The listing builds one solid part. Answer for the finished solid, in the listing's coordinates (mm). Face numbers are marked on the shaded views. Round coordinates to 2 decimals unless told otherwise and drop trailing zeros. Write each loop counter-clockwise with the first axis right and the second up, starting at its lowest first coordinate (ties: lowest second). Pieces come first, ordered by that corner, then holes.
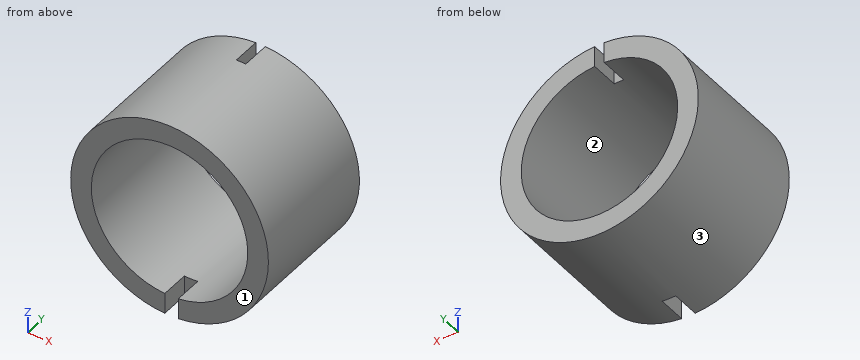
from build123d import *

# Parameters (mm, degrees)
SKETCH1_R           = 13.208
SKETCH1_R_2         = 10.45
BOSS_EXTRUDE1_DEPTH = 17.78
SKETCH2_W           = 1.27
SKETCH2_H           = 3.587114975
CUT_EXTRUDE1_DEPTH  = 3.81
SKETCH3_W           = 1.806448
SKETCH3_H           = 4.299301561
CUT_EXTRUDE2_DEPTH  = 3.81


with BuildPart() as part:
    # Sketch1 → Boss-Extrude1 (new body)
    with BuildSketch(Plane(origin=(0, 0, 0), x_dir=(1, 0, 0), z_dir=(0, 1, 0))):
        with Locations(Location((0, 0, 0), (0, 0, 270))):
            Circle(SKETCH1_R)
        with Locations(Location((0, 0, 0), (0, 0, 270))):
            Circle(SKETCH1_R_2, mode=Mode.SUBTRACT)
    extrude(amount=BOSS_EXTRUDE1_DEPTH)

    # Sketch2 → Cut-Extrude1 (cut)
    with BuildSketch(Plane(origin=(0, 17.78, 0), x_dir=(1, 0, 0), z_dir=(0, 1, 0))):
        with Locations((0, -11.851276013)):
            Rectangle(SKETCH2_W, SKETCH2_H)
    extrude(amount=-CUT_EXTRUDE1_DEPTH, mode=Mode.SUBTRACT)

    # Sketch3 → Cut-Extrude2 (cut)
    with BuildSketch(Plane.XZ):
        with Locations((0.268224, -12.348416978)):
            Rectangle(SKETCH3_W, SKETCH3_H)
    extrude(amount=-CUT_EXTRUDE2_DEPTH, mode=Mode.SUBTRACT)


solid = part.part
1. Section A-A on x = 0 is taken. Determine the outline of the cut face in (y, z), plus the area to 3 significant figures.
Geometry says:
outline: (0, 10.45) - (13.97, 10.45) - (13.97, 13.21) - (0, 13.21) - close; (3.81, -13.21) - (17.78, -13.21) - (17.78, -10.45) - (3.81, -10.45) - close
area: 77.1 mm2
2. Section C-C on z = -11 is taken. Determine the outline of the cut face in (x, y) (3 decimals).
Geometry says:
outline: (-7.311, 0) - (-0.635, 0) - (-0.635, 3.81) - (1.171, 3.81) - (1.171, 0) - (7.311, 0) - (7.311, 17.78) - (-7.311, 17.78) - close
3. Section B-B on z = 0 is taken. Determine the outline of the cut face in (x, y).
Geometry says:
outline: (-13.21, 0) - (-10.45, 0) - (-10.45, 17.78) - (-13.21, 17.78) - close; (10.45, 0) - (13.21, 0) - (13.21, 17.78) - (10.45, 17.78) - close
4. Given pin 1 (1.4 mm diameter, centred on y = 16, z = 11.5, fed in from +X); pin 2 (2 mm diameter, centred on y = 1, z = -12, fed in from -X); pin 3 (0.8 mm diameter, centred on y = 15.5, z = 11.5, fed in from -X), each flat-ended and moving along its own axis, determine where each tip first touches the part or whether it passes through.
Geometry says:
pin 1: stops at x = 7.6
pin 2: stops at x = -7.31
pin 3: stops at x = -7.16
5. For a pull along Z with two mould halves and no side action, classify the marked faces 1, 2 and 3 as released by +Z, released by -Z, zero draft, split by the parting line, or undercut.
Geometry says:
face 1: zero draft
face 2: undercut
face 3: split by the parting line
6. Straight lines are drawn through the part: line 1 along Z through (x, y) = (0, 13); line 2 along Z through (x, y) = (4.25, 10.75). For each, find the intervals that lie inside material, in ascending order.
Geometry says:
line 1: z = -13.21 to -10.45, 10.45 to 13.21
line 2: z = -12.51 to -9.55, 9.55 to 12.51
7. Section D-D on y = 13.25 is taken. Determine the outline of the cut face in (x, z).
Geometry says:
outline: circle Ø26.42 at (0, 0); hole circle Ø20.9 at (0, 0)
